Model file for the job. Use its own axes, mm. A direction names the side the tool comes from. Coordinates: 2 decimals unless noted, no trailing zeros. Order: outer loops, then holes, each group sorted by start corner. A loop starts at its lowest first (then second) coordinate and runs counter-clockwise, first axis right, second up. Notation, with made-up numbers: (-26.75, -25.75) -> (-15.75, -25.75) arc R14 ccw to (-15.75, 1.25) -> close; hole circle Ø1 at (-31, -4.5). An arc over 180 degrees is marked (long way). Use CSV: the item, a comma, the result in double quotes. Start each with the question number.
(1) Pull direction Y, two halves, no side cores. Call faces 4 (the flat face through (2, 0, 20.5)), 5 (the flat face through (-1.305, -0.74, 19.169)), 6 (the cylindrical face through (0, 5, 18)): pulls with the +Y half, pulls with the -Y half, needs draft (parallel to the pull), parting line crosses it, or undercut.
(2) Pin check, flat tips, straight feed: pin 1 Ø0.5 at (x, z) = (0.5, 19.5) entering from +Y; pin 2 Ø1.5 at (x, y) = (-3.5, 0) entering from -Z; pin 3 Ø3 at (y, z) = (-3.5, 10) entering from -X. Stop position of each tip, or through.
(3) Probe L1, parallel to Z at x = 2.25, y = 1.5; L2, parallel to Z at x = 3.75, y = -2; L3, parallel to Y at x = -0.25, z = 5.75. List the from-to ranges inside material, lowest first.
(4) Cut at A-A on x = 0. Write the cut outline in (y, z).
(5) Cut at B-B on z = 7. Write the cut outline in (x, y).
(6) Tool access for faces 1 (the flat face through (0, -1.5, 19)), 2 (the flat face through (0, 0, -9.5)), 3 (the cylindrical face through (-0.1, 2.5, -4.7)): list every direction of +Z, -Z, +X, -X, +Y, -Y with a clear straight run to the whole face (end or side of a thin tool).
```python
from build123d import *

# Parameters (mm, degrees)
CUT_EXTRUDE1_DEPTH = 2.7


with BuildPart() as part:
    # Sketch1 → Revolve1 (revolve)
    with BuildSketch(Plane(origin=(0, 0, 0), x_dir=(0, 0, -1), z_dir=(1, 0, 0)), mode=Mode.PRIVATE) as revolve1_sk:
        Polygon((-16, 3), (-16, 5), (-20, 5), (-20.5, 4.5), (-20.5, 0), (9.5, 0), (9.5, 2.5), (0, 2.5), (0, 3), align=None)
    revolve(revolve1_sk.sketch.rotate(Axis((0, 0, 5.584882278), (0, 0, -1)), 180), axis=Axis((0, 0, 5.584882278), (0, 0, -1)))

    # Sketch2 → Cut-Extrude1 (cut)
    with BuildSketch(Plane.XY.offset(20.5)):
        Polygon((0.866025404, -1.5), (1.732050808, 0), (0.866025404, 1.5), (-0.866025404, 1.5), (-1.732050808, 0), (-0.866025404, -1.5), align=None)
    extrude(amount=-CUT_EXTRUDE1_DEPTH, mode=Mode.SUBTRACT)


solid = part.part
```
Outcome:
1,face 4,"needs draft"
1,face 5,"undercut"
1,face 6,"parting line crosses it"
2,pin 1,"y = 4.99"
2,pin 2,"z = 0"
2,pin 3,"x = -2.24"
3,L1,"0 to 20.5"
3,L2,"16 to 20.5"
3,L3,"-2.99 to 2.99"
4,outline,"(-5, 16) -> (-3, 16) -> (-3, 0) -> (-2.5, 0) -> (-2.5, -9.5) -> (2.5, -9.5) -> (2.5, 0) -> (3, 0) -> (3, 16) -> (5, 16) -> (5, 20) -> (4.5, 20.5) -> (1.5, 20.5) -> (1.5, 17.8) -> (-1.5, 17.8) -> (-1.5, 20.5) -> (-4.5, 20.5) -> (-5, 20) -> close"
5,outline,"circle Ø6 at (0, 0)"
6,face 1,"+Z"
6,face 2,"-Z, +X, -X, +Y, -Y"
6,face 3,"-Z"
